from build123d import *
from build123d.topology import SkipClean

# Parameters (mm, degrees)
SKETCH_2_R          = 8
EXTRUDE_1_DEPTH     = 48
EXTRUDE_2_DEPTH     = 9
EXTRUDE_3_DEPTH     = 18
SKETCH_5_R          = 6
CUT_EXTRUDE_2_DEPTH = 20
EXTRUDE_START       = 20
SKETCH_6_R          = 10
SKETCH_6_R_2        = 6
EXTRUDE_6_DEPTH     = 20
SKETCH_1_R          = 8
CUT_EXTRUDE_4_DEPTH = 48


with BuildPart() as part:
    # 草图2 → 凸台-拉伸1 (new body)
    with BuildSketch(Plane(origin=(0, 0, 0), x_dir=(1, 0, 0), z_dir=(0, 1, 0))):
        with BuildLine():
            ThreePointArc((0, 16), (-6.92820323, 14.422205102), (-12.489995997, 10))
            ThreePointArc((-12.489995997, 10), (-16, 0), (-12.489995997, -10))
            ThreePointArc((-12.489995997, -10), (-6.92820323, -14.422205102), (0, -16))
            ThreePointArc((0, -16), (6.92820323, -14.422205102), (12.489995997, -10))
            ThreePointArc((12.489995997, -10), (16, 0), (12.489995997, 10))
            ThreePointArc((12.489995997, 10), (6.92820323, 14.422205102), (0, 16))
        make_face()
        with Locations(Location((0, 0, 0), (0, 0, 270))):
            Circle(SKETCH_2_R, mode=Mode.SUBTRACT)
    extrude(amount=EXTRUDE_1_DEPTH)

    # 草图3 → 凸台-拉伸2 (add)
    with BuildSketch(Plane(origin=(0, 0, 0), x_dir=(1, 0, 0), z_dir=(0, 1, 0))):
        with BuildLine():
            ThreePointArc((-33.361654635, 16), (-34.622558392, 13.049078527), (-35.623026261, 10))
            Line((-35.623026261, 10), (-12.489995997, 10))
            ThreePointArc((-12.489995997, 10), (-6.92820323, 14.422205102), (0, 16))
            Line((0, 16), (-33.361654635, 16))
        make_face()
        with BuildLine():
            ThreePointArc((0, -16), (-6.92820323, -14.422205102), (-12.489995997, -10))
            Line((-12.489995997, -10), (-35.623026261, -10))
            ThreePointArc((-35.623026261, -10), (-34.622558392, -13.049078527), (-33.361654635, -16))
            Line((-33.361654635, -16), (0, -16))
        make_face()
        with BuildLine():
            Line((33.361654635, 16), (0, 16))
            ThreePointArc((0, 16), (6.92820323, 14.422205102), (12.489995997, 10))
            Line((12.489995997, 10), (35.623026261, 10))
            ThreePointArc((35.623026261, 10), (34.622558392, 13.049078527), (33.361654635, 16))
        make_face()
        with BuildLine():
            ThreePointArc((12.489995997, -10), (6.92820323, -14.422205102), (0, -16))
            Line((0, -16), (33.361654635, -16))
            ThreePointArc((33.361654635, -16), (34.622558392, -13.049078527), (35.623026261, -10))
            Line((35.623026261, -10), (12.489995997, -10))
        make_face()
    extrude(amount=EXTRUDE_2_DEPTH)

    # 草图4 → 凸台-拉伸3 (add)
    with BuildSketch(Plane(origin=(0, 0, 0), x_dir=(1, 0, 0), z_dir=(0, 1, 0))):
        with BuildLine():
            Line((-12.489995997, 10), (-35.623026261, 10))
            ThreePointArc((-35.623026261, 10), (-36.22817767, 7.517921435), (-36.66060556, 5))
            Line((-36.66060556, 5), (-27, 5))
            ThreePointArc((-27, 5), (-22, 0), (-27, -5))
            Line((-27, -5), (-36.66060556, -5))
            ThreePointArc((-36.66060556, -5), (-36.22817767, -7.517921435), (-35.623026261, -10))
            Line((-35.623026261, -10), (-12.489995997, -10))
            ThreePointArc((-12.489995997, -10), (-16, 0), (-12.489995997, 10))
        make_face()
        with BuildLine():
            Line((35.623026261, 10), (12.489995997, 10))
            ThreePointArc((12.489995997, 10), (16, 0), (12.489995997, -10))
            Line((12.489995997, -10), (35.623026261, -10))
            ThreePointArc((35.623026261, -10), (36.22817767, -7.517921435), (36.66060556, -5))
            Line((36.66060556, -5), (27, -5))
            ThreePointArc((27, -5), (22, 0), (27, 5))
            Line((27, 5), (36.66060556, 5))
            ThreePointArc((36.66060556, 5), (36.22817767, 7.517921435), (35.623026261, 10))
        make_face()
    extrude(amount=EXTRUDE_3_DEPTH)

    # 草图5 → 切除-拉伸2 (cut, symmetric)
    with SkipClean():  # the faces are left unmerged after this step: merging them gives an invalid solid
        with BuildSketch(Plane.XY):
            with Locations((0, 28)):
                Circle(SKETCH_5_R)
        extrude(amount=CUT_EXTRUDE_2_DEPTH, both=True, mode=Mode.SUBTRACT)

    # 草图6 → 凸台-拉伸6 (add)
    with SkipClean():  # the faces are left unmerged after this step: merging them gives an invalid solid
        with BuildSketch(Plane.XY.offset(EXTRUDE_START)):
            with Locations(Location((0, 28, 0), (0, 0, 180))):
                Circle(SKETCH_6_R)
            with Locations(Location((0, 28, 0), (0, 0, 90))):
                Circle(SKETCH_6_R_2, mode=Mode.SUBTRACT)
        extrude(amount=-EXTRUDE_6_DEPTH)

    # 草图1 → 切除-拉伸4 (cut)
    with SkipClean():  # the faces are left unmerged after this step: merging them gives an invalid solid
        with BuildSketch(Plane(origin=(0, 0, 0), x_dir=(1, 0, 0), z_dir=(0, 1, 0))):
            with Locations(Location((0, 0, 0), (0, 0, 270))):
                Circle(SKETCH_1_R)
        extrude(amount=CUT_EXTRUDE_4_DEPTH, mode=Mode.SUBTRACT)


solid = part.part
Model file for the job. Use its own axes, mm. A direction names the side the tool comes from. Give positions to 0.01 mm unless a question says otherwise; leave off trailing zeros. Order: outer loops, then holes, each group sorted by start corner. A loop starts at its lowest first (then second) coordinate and runs counter-clockwise, first axis right, second up. Notation, with made-up numbers: (-17, -12) - (-9, -12) arc R14 cw to (-9, 0) - close; hole circle Ø2 at (45.5, -31.75). An arc over 180 degrees is marked (long way). Write item = value, one per line. Start each with the question number.
1. Cut at B-B, the plane z = 0. List the corners of the cut face in (x, y), and give its area (3 significant figures).
2. Cut at A-A, the plane y = 43.5. List the corners of the cut face in (x, z), and give its area (3 significant figures).
3. Drop flat-ended pins along their axis: P1, Ø10, axis at x = 28.5, z = -1.5, coming from the +Y side; P2, Ø4, axis at y = 39.5, z = -9.5, coming from the -X side; P3, Ø7.5, axis at x = -30.5, y = 13, coming from the -Z side; P4, Ø9.5, axis at x = 0, y = 28, coming from the -Z side. Give the stop position or say it passes through.
4. Probe line 1 along X through (y, z) = (36, 0); line 2 along Z through (x, y) = (27, 14); line 3 along Y through (x, z) = (17.5, 4.5). List the from-to ranges inside material, lowest first.
5. Cut at C-C, the plane x = 4. List the corners of the cut face in (y, z).
6. Which spindle directions (+Z, -Z, +X, -X, +Y, -Y) get a long thin tool onto all of the face, cutting with end or side? Do faces 4 (the flat face through (32, 9, -5)), 5 (the flat face through (-32, 9, 5)), 6 (the flat face through (-22, 9, -13)). Say none if no direction does.
7. Cut at D-D, the plane x = 26. List the corners of the cut face in (y, z), and give its area (3 significant figures).
8. Two-plate mould, pull along X, no slides. Class faces 1 (the flat face through (-9, 0, 0)), 2 (the cylindrical face through (22, 9, 0)), 3 (the cylindrical face through (3.226, 33.059, -10.571)): pulls with the +X half, pulls with the -X half, needs draft (parallel to the pull), parting line crosses it, or undercut.
Taken from the geometry:
q1.outline = (-22, 0) - (-8, 0) - (-8, 48) - (-16, 48) - (-16, 18) - (-22, 18) - close; (8, 0) - (22, 0) - (22, 18) - (16, 18) - (16, 48) - (8, 48) - close
q1.area = 984 mm²
q2.outline = circle Ø32 at (0, 0); hole circle Ø16 at (0, 0)
q2.area = 603 mm²
q3.P1 = 18
q3.P2 = -14.13
q3.P3 = -10
q3.P4 = through
q4.line_1 = -16 to -8, 8 to 16
q4.line_2 = -10 to -5, 5 to 10
q4.line_3 = 0 to 18
q5.outline = (0, -16) - (9, -16) - (9, -15.49) - (23.53, -15.49) - (23.53, -6.93) - (0, -6.93) - close; (0, 6.93) - (23.53, 6.93) - (23.53, 20) - (18.83, 20) - (18.83, 15.49) - (9, 15.49) - (9, 16) - (0, 16) - close; (32.47, -15.49) - (48, -15.49) - (48, -6.93) - (32.47, -6.93) - close; (32.47, 6.93) - (48, 6.93) - (48, 15.49) - (37.17, 15.49) - (37.17, 20) - (32.47, 20) - close
q6.face_4 = +X, +Y, -Y
q6.face_5 = -X, +Y, -Y
q6.face_6 = -Z, -X, +Y
q7.outline = (0, -16) - (9, -16) - (9, -10) - (18, -10) - (18, -4.9) - (0, -4.9) - close; (0, 4.9) - (18, 4.9) - (18, 10) - (9, 10) - (9, 16) - (0, 16) - close
q7.area = 292 mm²
q8.face_1 = needs draft
q8.face_2 = pulls with the +X half
q8.face_3 = undercut
